from build123d import *

# Parameters (mm, degrees)
SKETCH1_R                  = 11.1125
SKETCH1_R_2                = 13.5
BOSS_EXTRUDE1_DEPTH        = 3.175
M4_CLEARANCE_HOLE1_D       = 4.5
F_3_8_0_3750_DOWEL_HOLE1_D = 9.525


with BuildPart() as part:
    # Sketch1 → Boss-Extrude1 (new, symmetric)
    with BuildSketch(Plane(origin=(0, 0, 0), x_dir=(0, 0, -1), z_dir=(1, 0, 0))):
        with BuildLine():
            Line((104.098699929, 28.972456546), (0, 15))
            ThreePointArc((0, 15), (-2.052648501, 14.858890744), (-4.066677309, 14.438217884))
            ThreePointArc((-4.066677309, 14.438217884), (-14.858890744, -2.052648501), (0, -15))
            Line((0, -15), (106.075609583, -29.237803609))
            ThreePointArc((106.075609583, -29.237803609), (136.491140548, -12.979579055), (130.699290202, 21.018786481))
            ThreePointArc((130.699290202, 21.018786481), (119.340095093, 27.982362725), (106.075609583, 29.237803609))
            Line((106.075609583, 29.237803609), (105.337220563, 29.1386947))
            ThreePointArc((105.337220563, 29.1386947), (104.721310863, 29.030612592), (104.098699929, 28.972456546))
        make_face()
        Circle(SKETCH1_R, mode=Mode.SUBTRACT)
        with Locations((110, 0)):
            Circle(SKETCH1_R_2, mode=Mode.SUBTRACT)
    extrude(amount=BOSS_EXTRUDE1_DEPTH, both=True)

    # M4 Clearance Hole1 (through all)
    with Locations(Plane(origin=(3.175, 0, 0), x_dir=(0, 0, -1), z_dir=(1, 0, 0))):
        with Locations((99.25, 18.619546181), (131.5, 0), (99.25, -18.619546181)):
            Hole(M4_CLEARANCE_HOLE1_D / 2)

    # 3/8 (0.3750) Dowel Hole1 (through all)
    with Locations(Plane(origin=(3.175, 0, 0), x_dir=(0, 0, -1), z_dir=(1, 0, 0))):
        with Locations((65, 0)):
            Hole(F_3_8_0_3750_DOWEL_HOLE1_D / 2)


solid = part.part
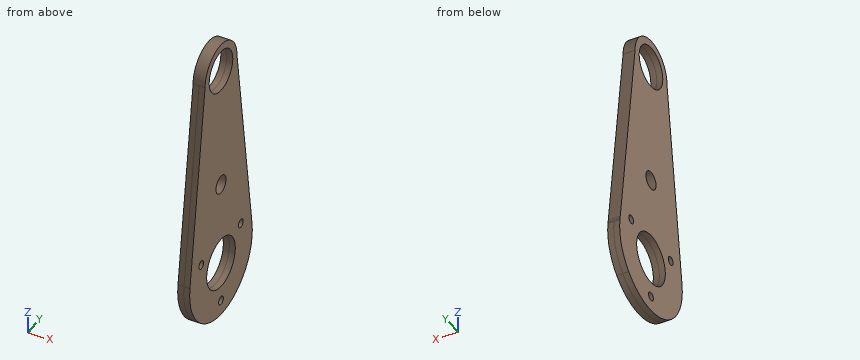
Input: part model. Units: mm. Frame: model coordinates. Give positions to 0.01 mm unless a question says otherwise; leave off trailing zeros. Write each loop counter-clockwise with the first axis right and the second up, starting at its lowest first coordinate (ties: lowest second). Pieces come first, ordered by that corner, then holes. Notation, with made-up numbers: M -31.5,72.25 L 12.5,72.25 A4 ccw 12.5,77.25 Z; hole C -27,-3.5 d1. An arc over 180 degrees is marked long. Write item = value, one per line. Start each with the question number.
1) Cut plane C-C on x = 1.5. Count the separate pieces of the cut face and the enclosed holes in it, then the cut area to 3 significant figures.
2) Cut plane D-D on z = -14.5. Return the cut outline in (x, y) (3 decimals), then the cut area to 3 significant figures.
3) Cut plane B-B on z = -99.25. Return the cut outline in (x, y) (3 decimals).
4) First-contact query: pin 1 Ø11 at (y, z) = (0, -65) entering from -X (3 decimals); pin 2 Ø2.5 at (y, z) = (-18.62, -99.25) entering from -X; pin 3 Ø3 at (x, z) = (-1.5, -38) entering from -Y; pin 4 Ø2 at (x, y) = (-2.5, 12.5) entering from -Z. Flat tips, straight axial feed; report the tip coordinate or a pass-through.
5) Cut plane A-A on z = -62. Return the cut outline in (x, y) (3 decimals), then the cut area to 3 significant figures.
6) Material intervals for line 1 along Z through (x, y) = (2, 7); line 2 along Y through (x, z) = (-2.45, -110); line 3 along Z through (x, y) = (1.5, 1), sorted ascending. Write a range as [from, to].
Solved:
q1.separate_pieces = 1
q1.enclosed_holes = 6
q1.area = 5,560 mm2
q2.outline = M -3.175,-16.946 L 3.175,-16.946 L 3.175,16.946 L -3.175,16.946 Z
q2.area = 215 mm2
q3.outline = M -3.175,-28.322 L 3.175,-28.322 L 3.175,-20.87 L -3.175,-20.87 Z; M -3.175,-16.37 L 3.175,-16.37 L 3.175,-8.166 L -3.175,-8.166 Z; M -3.175,8.166 L 3.175,8.166 L 3.175,16.37 L -3.175,16.37 Z; M -3.175,20.87 L 3.175,20.87 L 3.175,28.322 L -3.175,28.322 Z
q4.pin_1 = -3.175
q4.pin_2 = through
q4.pin_3 = -20.3
q4.pin_4 = -137.17
q5.outline = M -3.175,-23.322 L 3.175,-23.322 L 3.175,-3.699 L -3.175,-3.699 Z; M -3.175,3.699 L 3.175,3.699 L 3.175,23.322 L -3.175,23.322 Z
q5.area = 249 mm2
q6.line_1 = [-138.66, -121.54], [-98.46, -8.63], [8.63, 13.27]
q6.line_2 = [-29.5, -13.5], [13.5, 29.5]
q6.line_3 = [-139.48, -133.52], [-129.48, -123.46], [-96.54, -69.66], [-60.34, -11.07], [11.07, 14.97]
